Work out the finished part from the listing and answer in its coordinate system (mm). Give positions to 0.01 mm unless a question says otherwise; leave off trailing zeros. Loops run counter-clockwise (first coordinate to the right, second up) from the corner with the lowest first, then second, coordinate; pieces in that order, holes last. Notation, with made-up numbers: (-33, -1) - (24, -1) arc R26 cw to (24, 25) - close; hole circle Ø9 at (57, 81). An arc over 180 degrees is marked (long way). One line per question, with ' | ' between items. Start each with the question number.
1. Find the intervals of material crossed by line 1 (Y direction, x = 0, z = 22); line 2 (X direction, y = -4.5, z = 41.5); line 3 (Y direction, x = 3.75, z = 31.5), in increasing order.
2. For a pull along X with two mould halves and no side action, classify faces 1 (the face through (6, 0, 26)), 2 (the face through (-1.009, -7.684, 26.08)), 3 (the face through (4, -5, 0)) as released by +X, released by -X, zero draft, split by the parting line, or undercut.
3. Section C-C (z = 31.5) is taken. Determine the outline of the cut face in (x, y).
4. Each of these flat-tipped pins is pushed along its axis until it touches: pin 1 (1 mm diameter, centred on x = -2, z = 45.5, fed in from +Y); pin 2 (3 mm diameter, centred on y = 5.5, z = 12, fed in from -X); pin 3 (3 mm diameter, centred on x = 2, y = -3.5, fed in from +Z); pin 4 (4 mm diameter, centred on y = -2.5, z = 5.5, fed in from -X). Where does it stop, or does it pass through?
5. Section A-A (x = 0) is taken. Determine the outline of the cut face in (y, z), plus the area to 3 significant figures.
6. Section D-D (y = -7) is taken. Determine the outline of the cut face in (x, z), plus the area to 3 significant figures.
Autodesk Fusion 360 part; units mm, degrees
sketch "Sketch1" plane through (0, 0, 0) normal (0, 0, 1) x (1, 0, 0)
  circle A0 centre (0, 0) radius 7.75
  dimension "d1" = 15.5
extrude "Extrude1" add sketch "Sketch1" along normal blind 27.9
sketch "Sketch2" plane through (0, 0, 27.9) normal (0, 0, 1) x (-1, 0, 0)
  circle A0 centre (0, 0) radius 7.75
  circle A1 centre (0, 0) radius 6
  dimension "d4" = 12
extrude "Extrude2" cut sketch "Sketch2" against normal blind 30 contours A1
extrude "Extrude3" add 1 faces at (7.1155, -0.6831, 27.9) along direction (0, 0, 1) blind 15
extrude "Extrude4" add 1 faces at (7.1155, -0.6831, 42.9) along direction (0, 0, 1) blind 10
Conclusion:
1) line 1: -7.75 to -6, 6 to 7.75 | line 2: -6.31 to -3.97, 3.97 to 6.31 | line 3: -6.78 to -4.68, 4.68 to 6.78
2) face 1: undercut | face 2: split by the parting line | face 3: zero draft
3) outline: circle Ø15.5 at (0, 0); hole circle Ø12 at (0, 0)
4) pin 1: y = 7.6 | pin 2: x = -6.64 | pin 3: through | pin 4: x = -7.73
5) outline: (-7.75, 0) - (-6, 0) - (-6, 52.9) - (-7.75, 52.9) - close; (6, 0) - (7.75, 0) - (7.75, 52.9) - (6, 52.9) - close | area: 185 mm²
6) outline: (-3.33, 0) - (3.33, 0) - (3.33, 52.9) - (-3.33, 52.9) - close | area: 352 mm²
